```python
from build123d import *

# Parameters (mm, degrees)
CROQUIS2_W              = 240
CROQUIS2_H              = 140
SALIENTE_EXTRUIR1_DEPTH = 10
CROQUIS3_R              = 1.6
CROQUIS3_W              = 20
CROQUIS3_H              = 6.5
CROQUIS3_W_2            = 10.16
CROQUIS3_H_2            = 8.96
CORTAR_EXTRUIR1_DEPTH   = 279.028775489
MATRIZL1_COUNT          = 3
MATRIZL1_PITCH          = 70
MATRIZL1_COUNT_DIR2     = 2
MATRIZL1_PITCH_DIR2     = 70


with BuildPart() as part:
    # Croquis2 → Saliente-Extruir1 (new body)
    with BuildSketch(Plane.YZ):
        with Locations((120, 70)):
            Rectangle(CROQUIS2_W, CROQUIS2_H)
    extrude(amount=SALIENTE_EXTRUIR1_DEPTH)

    # Croquis3 → Cortar-Extruir1 (cut, symmetric)
    with BuildSketch(Plane.YZ.offset(10)):
        with Locations(Location((30, 125, 0), (0, 0, 270))):
            Circle(CROQUIS3_R)
        with Locations(Location((30, 85, 0), (0, 0, 270))):
            Circle(CROQUIS3_R)
        with Locations((55.75, 126.25)):
            Rectangle(CROQUIS3_W, CROQUIS3_H)
        with Locations((59.11, 85)):
            Rectangle(CROQUIS3_W_2, CROQUIS3_H_2)
    cortar_extruir1 = extrude(amount=CORTAR_EXTRUIR1_DEPTH, both=True, mode=Mode.SUBTRACT)

    # MatrizL1: Cortar-Extruir1 3 × 2
    with Locations(*[(0, i * MATRIZL1_PITCH, -j * MATRIZL1_PITCH_DIR2) for i in range(MATRIZL1_COUNT) for j in range(MATRIZL1_COUNT_DIR2) if (i, j) != (0, 0)]):
        add(cortar_extruir1, mode=Mode.SUBTRACT)


solid = part.part
```
Could you check a few things on this model? Use its own coordinates, in mm. A direction names the side the tool comes from. Give positions to 0.01 mm unless a question says otherwise; leave off trailing zeros. Loops run counter-clockwise (first coordinate to the right, second up) from the corner with the lowest first, then second, coordinate; pieces in that order, holes last. Notation, with made-up numbers: (36.5, -4) - (91.5, -4) arc R19 ccw to (91.5, 32) - close; hole circle Ø7 at (-25.5, -7). An arc over 180 degrees is marked (long way). Answer in a Markdown table with one row per item. Add a question column.
Q1. Please list where this line runs through material, in increasing order: L1, parallel to Z at x = 1.5, y = 194.5. Write a range as from..to.
Q2. Which directions (+Z, -Z, +X, -X, +Y, -Y) give clear straight access to the entire face, cutting with the end or side of a thin tool? Please do faces 3 (the face through (5, 124.03, 15)), 4 (the face through (10, 118, 71)).
Q3. For pin 1 (2.5 mm diameter, centred on y = 30, z = 15, fed in from -X), with a flat end and sliding along its axis, tell me the tip position at first contact or that it passes through.
Q4. We'd pull the mould along Z, two halves only. Please class faces 1 (the face through (5, 240, 69)), 2 (the face through (5, 59, 89.48)): +Z half, -Z half, draft (parallel to the pull), parting line (faces both ways), or undercut.
Q5. If we section it at A-A (y = 49.5): List the corners of the cut face in (x, z) for me.
Q6. If we section it at B-B (x = 4.5): State how many separate pieces and enclosed holes the cut face has, plus the area to 3 significant figures.
The answers:
| question | item | result |
|---|---|---|
| 1 | L1 | z = 0..10.52, 19.48..53, 59.5..80.52, 89.48..123, 129.5..140 |
| 2 | face 3 | +X, -X |
| 2 | face 4 | +Z, -Z, +X, +Y, -Y |
| 3 | pin 1 | passes through |
| 4 | face 1 | draft |
| 4 | face 2 | undercut |
| 5 | outline | (0, 0) - (10, 0) - (10, 53) - (0, 53) - close; (0, 59.5) - (10, 59.5) - (10, 123) - (0, 123) - close; (0, 129.5) - (10, 129.5) - (10, 140) - (0, 140) - close |
| 6 | separate pieces | 1 |
| 6 | enclosed holes | 24 |
| 6 | area | 32,200 mm^2 |
